Autodesk Inventor part; units mm, degrees
ref_plane "YZ Plane" through (0, 0, 0) normal (1, 0, 0) x (0, 1, 0)
ref_plane "XZ Plane" through (0, 0, 0) normal (0, 1, 0) x (-1, 0, 0)
ref_plane "XY Plane" through (0, 0, 0) normal (0, 0, 1) x (1, 0, 0)
sketch "Boceto1" plane through (0, 0, 0) normal (0, 1, 0) x (-1, 0, 0)
  circle A0 centre (28.5, 0) radius 1.5
  circle A1 centre (28.5, -8) radius 1.5
  circle A2 centre (28.5, 8) radius 1.5
  circle A3 centre (36.5, 0) radius 1.5
  circle A4 centre (20.5, 0) radius 1.5
  circle A5 centre (28.5, 0) radius 47.5
  line L0 (57, 33) -> (43, 33)
  line L1 (43, 33) -> (43, 30)
  line L2 (35.5, 30) -> (35.5, 33)
  line L3 (35.5, 33) -> (21.5, 33)
  line L4 (21.5, 33) -> (21.5, 30)
  line L5 (14, 30) -> (14, 33)
  line L6 (14, 33) -> (0, 33)
  line L7 (43, 30) -> (57, 30)
  line L8 (21.5, 30) -> (35.5, 30)
  line L9 (14, 30) -> (0, 30)
  line L10 (0, 30) -> (0, 33)
  line L11 (57, 33) -> (57, 30)
  line L12 (35.5, -30) -> (35.5, -33)
  line L13 (21.5, -30) -> (35.5, -30)
  line L14 (35.5, -33) -> (21.5, -33)
  line L15 (21.5, -33) -> (21.5, -30)
  line L16 (57, -33) -> (43, -33)
  line L17 (43, -33) -> (43, -30)
  line L18 (43, -30) -> (57, -30)
  line L19 (14, -30) -> (14, -33)
  line L20 (14, -30) -> (0, -30)
  line L21 (14, -33) -> (0, -33)
  line L22 (0, -30) -> (0, -33)
  line L23 (57, -33) -> (57, -30)
extrude "Extrusión1" add sketch "Boceto1" along normal blind 3
sketch "Boceto2" plane through (-28.5, 0, 0) normal (0, -1, 0) x (1, 0, 0)
  circle A0 centre (0, 0) radius 3.5
  point P0 (28.5, 0)
  dimension "d23" = 7
extrude "Extrusión2" cut sketch "Boceto2" against normal blind 10
sketch "Boceto3" plane through (-28.5, 0, 0) normal (0, -1, 0) x (1, 0, 0)
  circle A0 centre (0, 0) radius 4.5
  point P0 (28.5, 0)
  dimension "d26" = 9
extrude "Extrusión3" cut sketch "Boceto3" against normal blind 10
sketch "Boceto4" plane through (-28.5, 0, 0) normal (0, -1, 0) x (1, 0, 0)
  line L0 (-40.25, 9.75) -> (9.75, 9.75)
  line L1 (9.75, 9.75) -> (9.75, -9.75)
  line L2 (9.75, -9.75) -> (-40.25, -9.75)
  line L3 (-40.25, -9.75) -> (-40.25, 9.75)
  circle A0 centre (-43.5, 4.875) radius 1.5
  circle A1 centre (-43.5, -4.875) radius 1.5
  circle A2 centre (13, 4.875) radius 1.5
  circle A3 centre (13, -4.875) radius 1.5
  point P0 (28.5, 0)
  point P1 (-28.5, 33)
  point P2 (28.5, 33)
  point P3 (28.5, 30)
  point P4 (-28.5, -33)
  point P5 (0, 0)
  dimension "d32" = 50
extrude "Extrusión4" cut sketch "Boceto4" against normal blind 3
sketch "Boceto5" plane through (-28.5, 0, 0) normal (0, -1, 0) x (1, 0, 0)
  point P0 (28.5, 0)
  point P1 (-14.5, 33)
  point P2 (-28.5, 33)
  point P3 (7, 33)
  point P4 (-7, 33)
properties part number "base2"
For this review, take the finished solid that the model builds, in its own axes (mm). Give positions to 0.01 mm unless a question says otherwise; leave off trailing zeros. Loops run counter-clockwise (first coordinate to the right, second up) from the corner with the lowest first, then second, coordinate; pieces in that order, holes last. Notation, with made-up numbers: M 61.5,4.25 L 76.5,4.25 A30 ccw 76.5,26.25 Z; hole C -1.5,11.5 d1. An arc over 180 degrees is marked long. Put each result on its own line as item: value. Start each with the question number.
(1) The part is to be moulded in two halves that separate along X. For faces 1 (the flat face through (0, 1, -31)), 2 (the flat face through (-28, 3, -10)), say which applies: +X half, -X half, draft (parallel to the pull), parting line (faces both ways), or undercut.
(2) For pin 1 (0.9 mm diameter, centred on y = 2, z = 31.5, fed in from +X); pin 2 (0.9 mm diameter, centred on y = 1, z = 32, fed in from +X); pin 3 (1.5 mm diameter, centred on x = 1.5, y = 0.5, fed in from +Z), all flat-tipped, find the tip position at first contact; note any pin that passes through.
(3) Add section C-C, the plane y = 1.55. Give the number of separate pieces and of enclosed holes in the cut face, then the cut area to 3 significant figures.
(4) Wall thickness on L1, parallel to Z at x = -29, y = 1.9; L2, parallel to Z at x = -72, y = 1.4 (3 decimals); L3, parallel to X at y = 1.2, z = 1.5: over which ranges is each line inside the solid? List them lowest first.
(5) Add section B-B, the plane z = 0. Write out the cut boundary in (x, y).
(6) Add section D-D, the plane x = -72. Write out the cut boundary in (y, z) (3 decimals).
(7) Add section A-A, the plane x = -28.5. Write out the cut boundary in (y, z).
Result:
1. face 1: undercut
1. face 2: draft
2. pin 1: stops at x = 7.45
2. pin 2: stops at x = 7.01
2. pin 3: stops at z = 37.43
3. separate pieces: 1
3. enclosed holes: 11
3. area: 5,830 mm^2
4. L1: z = -47.5 to -33, -30 to -9.75, 9.75 to 30, 33 to 47.5
4. L2: z = -19.079 to -6.375, -3.375 to 3.375, 6.375 to 19.079
4. L3: x = -75.98 to -68.75, -18.75 to 18.98
5. outline: M -76,0 L -68.75,0 L -68.75,3 L -76,3 Z; M -18.75,0 L 19,0 L 19,3 L -18.75,3 Z
6. outline: M 0,-19.079 L 3,-19.079 L 3,-6.375 L 0,-6.375 Z; M 0,-3.375 L 3,-3.375 L 3,3.375 L 0,3.375 Z; M 0,6.375 L 3,6.375 L 3,19.079 L 0,19.079 Z
7. outline: M 0,-47.5 L 3,-47.5 L 3,-33 L 0,-33 Z; M 0,-30 L 3,-30 L 3,-9.75 L 0,-9.75 Z; M 0,9.75 L 3,9.75 L 3,30 L 0,30 Z; M 0,33 L 3,33 L 3,47.5 L 0,47.5 Z
